from build123d import *

# Parameters (mm, degrees)
F1_W          = 44.45
F1_H          = 31.75
F2_DEPTH      = 6.985
F4_DEPTH      = 44.45
F6_DEPTH      = 15.24
F6_DEPTH_BACK = 15.24
F7_W          = 20
F7_H          = 8.0811108913
F8_DEPTH      = 25.4
F9_R          = 1.6
F10_DEPTH     = 25.4
F11_R         = 1.6
F12_DEPTH     = 5.7
F13_W         = 31.75
F13_H         = 1.5
F14_DEPTH     = 2
F14_TAPER     = 10
F15_F1_R      = 0.254
F15_F2_R      = 0.254
F16_R         = 5.08
F18_R         = 1.27
F19_T1_DEPTH  = 5.24
F19_T3_DEPTH  = 5.24
F19_T5_DEPTH  = 8.89
F19_T7_DEPTH  = 29.21
F19_T9_DEPTH  = 41.91
F19_S13_W     = 1.2954
F19_S13_H     = 1.2954
F19_T14_DEPTH = 1.2954
F19_S19_W     = 1.2954
F19_S19_H     = 1.2954
F19_T20_DEPTH = 1.2954
F19_S25_W     = 1.2954
F19_S25_H     = 1.2954
F19_T26_DEPTH = 1.2954
F19_S31_W     = 1.2954
F19_S31_H     = 1.2954
F19_T32_DEPTH = 1.2954


# Not quite as in the source:
# - a fillet or chamfer that OpenCascade refuses, or shapes differently, is made with other operations: its cross-section is extruded or revolved along the edge and cut away or added
# - a feature of the source that left no trace in its solid (it failed there, or was rolled back) is left out


with BuildPart() as f2:
    # F1 (on Top) → F2 (new body)
    with BuildSketch(Plane.XY):
        Rectangle(F1_W, F1_H)
    extrude(amount=-F2_DEPTH)

    # F3 (on face) → F4 (cut, through all)
    with BuildSketch(Plane.YZ.offset(22.225)):
        with BuildLine():
            add(Edge.make_bspline(
                [(-4.125, 4.125), (-2.4255892558, 4.1137489608), (-0.0276085061, 2.971292738), (2.5249406681, 4.1137612248), (4.191, 4.191)],
                knots=[0, 0, 0, 0, 0.4977710734, 1, 1, 1, 1], degree=3))
            ThreePointArc((-4.125, 4.125), (-7.0418154724, 2.9168154724), (-8.25, 0))
            ThreePointArc((-8.25, 0), (-7.0418154724, -2.9168154724), (-4.125, -4.125))
            add(Edge.make_bspline(
                [(-4.125, -4.125), (-2.9335741419, -4.2006121948), (0.4172014685, -3.0581585459), (2.1438994445, -4.2006121948), (4.191, -4.191)],
                knots=[0, 0, 0, 0, 0.497799261, 1, 1, 1, 1], degree=3))
            ThreePointArc((4.191, -4.191), (7.15448452, -2.96348452), (8.382, 0))
            ThreePointArc((8.382, 0), (7.15448452, 2.96348452), (4.191, 4.191))
        make_face()
    extrude(amount=-F4_DEPTH, mode=Mode.SUBTRACT)

    # F5 (on Right) → F6 (join, two sides)
    with BuildSketch(Plane.YZ) as f6_sk:
        with BuildLine():
            ThreePointArc((-31.115, -30.5349261659), (0, -16.985), (31.115, -30.5349261659))
            Line((31.115, -30.5349261659), (28.575, -25.0251942949))
            ThreePointArc((28.575, -25.0251942949), (19.6900567688, -18.8213349574), (9.525, -15.0661108913))
            ThreePointArc((9.525, -15.0661108913), (0, -13.985), (-9.525, -15.0661108913))
            ThreePointArc((-9.525, -15.0661108913), (-19.6900567688, -18.8213349574), (-28.575, -25.0251942949))
            Line((-28.575, -25.0251942949), (-31.115, -30.5349261659))
        make_face()
        with BuildLine():
            ThreePointArc((-9.525, -15.0661108913), (0, -13.985), (9.525, -15.0661108913))
            Line((9.525, -15.0661108913), (9.525, -6.985))
            Line((9.525, -6.985), (-9.525, -6.985))
            Line((-9.525, -6.985), (-9.525, -15.0661108913))
        make_face()
    extrude(amount=F6_DEPTH)
    extrude(f6_sk.sketch, amount=-F6_DEPTH_BACK)

    # F7 (on face) → F8 (cut)
    with BuildSketch(Plane.XZ.offset(9.525)):
        with Locations((0, -11.0255554456)):
            Rectangle(F7_W, F7_H)
    extrude(amount=-F8_DEPTH, mode=Mode.SUBTRACT)

    # F9 (on face) → F10 (cut)
    with BuildSketch(Plane(origin=(0, 0, -6.985), x_dir=(1, 0, 0), z_dir=(0, 0, -1))):
        with Locations((-18.669, 12.319)):
            Circle(F9_R)
        with Locations((18.669, -12.319)):
            Circle(F9_R)
    extrude(amount=-F10_DEPTH, mode=Mode.SUBTRACT)

    # F11 (on face) → F12 (cut)
    with BuildSketch(Plane(origin=(0, 0, -6.985), x_dir=(1, 0, 0), z_dir=(0, 0, -1))):
        Polygon((-17.344, 10.02403268), (-16.019, 12.319), (-17.344, 14.61396732), (-19.994, 14.61396732), (-21.319, 12.319), (-19.994, 10.02403268), align=None)
        with Locations((-18.669, 12.319)):
            Circle(F11_R, mode=Mode.SUBTRACT)
        Polygon((19.994, -14.61396732), (21.319, -12.319), (19.994, -10.02403268), (17.344, -10.02403268), (16.019, -12.319), (17.344, -14.61396732), align=None)
        with Locations((18.669, -12.319)):
            Circle(F11_R, mode=Mode.SUBTRACT)
    extrude(amount=-F12_DEPTH, mode=Mode.SUBTRACT)

    # F13 (on face) → F14 (join)
    with BuildSketch(Plane.XY):
        with Locations((-4.35, 13.125)):
            Rectangle(F13_W, F13_H)
        with Locations((4.35, -13.125)):
            Rectangle(F13_W, F13_H)
    extrude(amount=F14_DEPTH, taper=F14_TAPER)

    # F15: fillet of radius 0.254 on 2 edges, made by hand

    # F15_f1
    f15_f1_edges = [f2.edges().sort_by_distance(p)[0] for p in [
        (0, -31.115, -30.5349261659),
    ]]
    fillet(f15_f1_edges, radius=F15_F1_R)

    # F15_f2
    f15_f2_edges = [f2.edges().sort_by_distance(p)[0] for p in [
        (0, 31.115, -30.5349261659),
    ]]
    fillet(f15_f2_edges, radius=F15_F2_R)

    # F16
    f16_edges = [f2.edges().sort_by_distance(p)[0] for p in [
        (0, 28.575, -25.025194),
        (0, -28.575, -25.025194),
    ]]
    fillet(f16_edges, radius=F16_R)

    # F18
    f18_edges = [f2.edges().sort_by_distance(p)[0] for p in [
        (12.62, 9.525, -6.985),
        (15.24, 0, -6.985),
        (12.62, -9.525, -6.985),
        (10, 0, -6.985),
        (-12.62, -9.525, -6.985),
        (-15.24, 0, -6.985),
        (-10, 0, -6.985),
        (-12.62, 9.525, -6.985),
    ]]
    fillet(f18_edges, radius=F18_R)

    # F19: fillet of radius 1.27 on 12 edges, made by hand

    # F19_s2 → F19_t1 (join)
    with BuildSketch(Plane.YZ.offset(-15.24)):
        with BuildLine():
            ThreePointArc((9.525, -14.0670689448), (9.7923311345, -14.8465271838), (10.4817797578, -15.2978382489))
            ThreePointArc((10.4817797578, -15.2978382489), (10.0040608486, -15.1792042016), (9.525, -15.0661108913))
            Line((9.525, -15.0661108913), (9.525, -14.0670689448))
        make_face()
        with BuildLine():
            ThreePointArc((-9.525, -14.0670689448), (-9.7923311345, -14.8465271838), (-10.4817797578, -15.2978382489))
            ThreePointArc((-10.4817797578, -15.2978382489), (-10.0040608486, -15.1792042016), (-9.525, -15.0661108913))
            Line((-9.525, -15.0661108913), (-9.525, -14.0670689448))
        make_face()
    extrude(amount=F19_T1_DEPTH)

    # F19_s4 → F19_t3 (join)
    with BuildSketch(Plane.YZ.offset(10)):
        with BuildLine():
            ThreePointArc((10.4817797578, -15.2978382489), (9.7923311345, -14.8465271838), (9.525, -14.0670689448))
            Line((9.525, -14.0670689448), (9.525, -15.0661108913))
            ThreePointArc((9.525, -15.0661108913), (10.0040608486, -15.1792042016), (10.4817797578, -15.2978382489))
        make_face()
        with BuildLine():
            ThreePointArc((-10.4817797578, -15.2978382489), (-9.7923311345, -14.8465271838), (-9.525, -14.0670689448))
            Line((-9.525, -14.0670689448), (-9.525, -15.0661108913))
            ThreePointArc((-9.525, -15.0661108913), (-10.0040608486, -15.1792042016), (-10.4817797578, -15.2978382489))
        make_face()
    extrude(amount=F19_T3_DEPTH)

    # F19_s6 → F19_t5 (cut)
    with BuildSketch(Plane.XY.offset(-5.715)):
        with BuildLine():
            ThreePointArc((-20.955, -15.875), (-21.8530256121, -15.5030256121), (-22.225, -14.605))
            Line((-22.225, -14.605), (-22.225, -15.875))
            Line((-22.225, -15.875), (-20.955, -15.875))
        make_face()
        with BuildLine():
            ThreePointArc((22.225, -14.605), (21.8530256121, -15.5030256121), (20.955, -15.875))
            Line((20.955, -15.875), (22.225, -15.875))
            Line((22.225, -15.875), (22.225, -14.605))
        make_face()
        with BuildLine():
            ThreePointArc((22.225, 14.605), (21.8530256121, 15.5030256121), (20.955, 15.875))
            Line((20.955, 15.875), (22.225, 15.875))
            Line((22.225, 15.875), (22.225, 14.605))
        make_face()
        with BuildLine():
            ThreePointArc((-20.955, 15.875), (-21.8530256121, 15.5030256121), (-22.225, 14.605))
            Line((-22.225, 14.605), (-22.225, 15.875))
            Line((-22.225, 15.875), (-20.955, 15.875))
        make_face()
    extrude(amount=F19_T5_DEPTH, mode=Mode.SUBTRACT)

    # F19_s8 → F19_t7 (cut)
    with BuildSketch(Plane.XZ.offset(-14.605)):
        with BuildLine():
            ThreePointArc((-20.955, -6.985), (-21.8530256121, -6.6130256121), (-22.225, -5.715))
            Line((-22.225, -5.715), (-22.225, -6.985))
            Line((-22.225, -6.985), (-20.955, -6.985))
        make_face()
        with BuildLine():
            ThreePointArc((20.955, -6.985), (21.8530256121, -6.6130256121), (22.225, -5.715))
            Line((22.225, -5.715), (22.225, -6.985))
            Line((22.225, -6.985), (20.955, -6.985))
        make_face()
    extrude(amount=F19_T7_DEPTH, mode=Mode.SUBTRACT)

    # F19_s10 → F19_t9 (cut)
    with BuildSketch(Plane.YZ.offset(-20.955)):
        with BuildLine():
            ThreePointArc((-14.605, -6.985), (-15.5030256121, -6.6130256121), (-15.875, -5.715))
            Line((-15.875, -5.715), (-15.875, -6.985))
            Line((-15.875, -6.985), (-14.605, -6.985))
        make_face()
        with BuildLine():
            ThreePointArc((14.605, -6.985), (15.5030256121, -6.6130256121), (15.875, -5.715))
            Line((15.875, -5.715), (15.875, -6.985))
            Line((15.875, -6.985), (14.605, -6.985))
        make_face()
    extrude(amount=F19_T9_DEPTH, mode=Mode.SUBTRACT)


with BuildPart() as f19_tool12:
    # F19_s13 → F19_t14 (new body)
    with BuildSketch(Plane.YZ.offset(-20.955)):
        with Locations((-15.2527, -6.3627)):
            Rectangle(F19_S13_W, F19_S13_H)
    extrude(amount=-F19_T14_DEPTH)

    # F19_s15 → F19_t16 (revolve, cut)
    with BuildSketch(Plane(origin=(-20.955, -14.605, -5.715), x_dir=(0, 0.7071067812, 0.7071067812), z_dir=(0, -0.7071067812, 0.7071067812))):
        with BuildLine():
            ThreePointArc((0, -1.27), (1.27, 0), (0, 1.27))
            Line((0, 1.27), (0, -1.27))
        make_face()
    revolve(axis=Axis((-20.955, -14.605, -5.715), (-1, 0, 0)), mode=Mode.SUBTRACT)


with BuildPart() as f2_1:
    add(f2.part)

    # F19_t11: cut F19_tool12
    add(f19_tool12.part, mode=Mode.SUBTRACT)


with BuildPart() as f19_tool18:
    # F19_s19 → F19_t20 (new body)
    with BuildSketch(Plane.XY.offset(-5.715)):
        with Locations((-21.6027, 15.2527)):
            Rectangle(F19_S19_W, F19_S19_H)
    extrude(amount=-F19_T20_DEPTH)

    # F19_s21 → F19_t22 (revolve, cut)
    with BuildSketch(Plane(origin=(-20.955, 14.605, -5.715), x_dir=(0.7071067812, -0.7071067812, 0), z_dir=(0.7071067812, 0.7071067812, 0))):
        with BuildLine():
            ThreePointArc((0, -1.27), (1.27, 0), (0, 1.27))
            Line((0, 1.27), (0, -1.27))
        make_face()
    revolve(axis=Axis((-20.955, 14.605, -5.715), (0, 0, -1)), mode=Mode.SUBTRACT)


with BuildPart() as f2_2:
    add(f2_1.part)

    # F19_t17: cut F19_tool18
    add(f19_tool18.part, mode=Mode.SUBTRACT)


with BuildPart() as f19_tool24:
    # F19_s25 → F19_t26 (new body)
    with BuildSketch(Plane.XY.offset(-5.715)):
        with Locations((21.6027, -15.2527)):
            Rectangle(F19_S25_W, F19_S25_H)
    extrude(amount=-F19_T26_DEPTH)

    # F19_s27 → F19_t28 (revolve, cut)
    with BuildSketch(Plane(origin=(20.955, -14.605, -5.715), x_dir=(-0.7071067812, 0.7071067812, 0), z_dir=(-0.7071067812, -0.7071067812, 0))):
        with BuildLine():
            ThreePointArc((0, -1.27), (1.27, 0), (0, 1.27))
            Line((0, 1.27), (0, -1.27))
        make_face()
    revolve(axis=Axis((20.955, -14.605, -5.715), (0, 0, -1)), mode=Mode.SUBTRACT)


with BuildPart() as f2_3:
    add(f2_2.part)

    # F19_t23: cut F19_tool24
    add(f19_tool24.part, mode=Mode.SUBTRACT)


with BuildPart() as f19_tool30:
    # F19_s31 → F19_t32 (new body)
    with BuildSketch(Plane.XY.offset(-5.715)):
        with Locations((21.6027, 15.2527)):
            Rectangle(F19_S31_W, F19_S31_H)
    extrude(amount=-F19_T32_DEPTH)

    # F19_s33 → F19_t34 (revolve, cut)
    with BuildSketch(Plane(origin=(20.955, 14.605, -5.715), x_dir=(-0.7071067812, -0.7071067812, 0), z_dir=(0.7071067812, -0.7071067812, 0))):
        with BuildLine():
            ThreePointArc((0, -1.27), (1.27, 0), (0, 1.27))
            Line((0, 1.27), (0, -1.27))
        make_face()
    revolve(axis=Axis((20.955, 14.605, -5.715), (0, 0, -1)), mode=Mode.SUBTRACT)


with BuildPart() as f2_4:
    add(f2_3.part)

    # F19_t29: cut F19_tool30
    add(f19_tool30.part, mode=Mode.SUBTRACT)


solid = f2_4.part
Could you check a few things on this model? Use its own coordinates, in mm. A direction names the side the tool comes from. Round coordinates to 2 decimals unless told otherwise and drop trailing zeros. Order: outer loops, then holes, each group sorted by start corner. A loop starts at its lowest first (then second) coordinate and runs counter-clockwise, first axis right, second up. Notation, with made-up numbers: M 13,82 L 64,82 A15 ccw 64,89 Z; hole C 33.5,-21.75 d11. An arc over 180 degrees is marked long. One line per item, written item: value.
(1) Imagine slicing it at A-A (z = -11). Write out the boundary of the cut face in (x, y) (3 decimals).
Ans:
outline: M -15.24,-9.525 L -10,-9.525 L -10,9.525 L -15.24,9.525 Z; M 10,-9.525 L 15.24,-9.525 L 15.24,9.525 L 10,9.525 Z
(2) I need wall thicknesses on line 1 along X through (y, z) = (-18.5, -20); line 2 along Y through (x, z) = (6.5, -21); line 3 along X through (y, z) = (4, -8). Which ranges of each line are inside material? Lowest first, please. Write a range as from..to.
Ans:
line 1: x = -15.24..15.24
line 2: y = -23.39..-18.03, 18.03..23.39
line 3: x = -15.27..-9.97, 9.97..15.27
(3) Which directions (+Z, -Z, +X, -X, +Y, -Y) give clear straight access to the entire face, cutting with the end or side of a thin tool? Please do faces 1 (the cylindrical face through (-12.657, -9.785, -14.837)), 2 (the flat face through (15.24, 0, -16)), 3 (the cylindrical face through (0.31, 7.12, -3)), 4 (the flat face through (0, 0, -15.066)), 5 (the flat face through (-19, -14.614, -4)).
Ans:
face 1: +X, -X, -Y
face 2: -Z, +X, +Y, -Y
face 3: +Z, +X, -X
face 4: +Y, -Y
face 5: -Z
(4) Imagine slicing it at B-B (z = -2.5). Write out the boundary of the cut face in (x, y) (3 decimals).
Ans:
outline: M -22.225,-14.605 A1.27 ccw -20.955,-15.875 L 20.955,-15.875 A1.27 ccw 22.225,-14.605 L 22.225,-7.406 L -22.225,-7.406 Z; M -22.225,7.555 L 22.225,7.555 L 22.225,14.605 A1.27 ccw 20.955,15.875 L -20.955,15.875 A1.27 ccw -22.225,14.605 Z; hole M -21.319,-12.319 L -19.994,-14.614 L -17.344,-14.614 L -16.019,-12.319 L -17.344,-10.024 L -19.994,-10.024 Z; hole M 16.019,12.319 L 17.344,10.024 L 19.994,10.024 L 21.319,12.319 L 19.994,14.614 L 17.344,14.614 Z
(5) I'm going to push flat-ended pins straight in: P1, Ø14.5, axis at x = -7, y = 3.5, coming from the -Z side; P2, Ø2, axis at x = -19, z = -3.5, coming from the -Y side (3 decimals); P3, Ø8, axis at x = -12.5, y = 24, coming from the +Z side (3 decimals); P4, Ø2, axis at y = -1, z = -19, coming from the -X side. Where does each tip first touch, or does it pass through?
Ans:
P1: stops at z = -18.37
P2: stops at y = -15.875
P3: stops at z = -18.985
P4: passes through
(6) Imagine slicing it at C-C (y = -5.5). Write out the boundary of the cut face in (x, z) (3 decimals).
Ans:
outline: M -22.225,-5.715 A1.27 ccw -20.955,-6.985 L -16.51,-6.985 A1.27 cw -15.24,-8.255 L -15.24,-17.342 L 15.24,-17.342 L 15.24,-8.255 A1.27 cw 16.51,-6.985 L 20.955,-6.985 A1.27 ccw 22.225,-5.715 L 22.225,-3.889 L -22.225,-3.889 Z; hole M -10,-15.066 L 10,-15.066 L 10,-8.255 A1.27 ccw 8.73,-6.985 L -8.73,-6.985 A1.27 ccw -10,-8.255 Z
(7) If we mould it in two halves opening along Z, with no side actions, what happens to faces 6 (the flat face through (-16.7, -13.5, -4.2)), 7 (the flat face through (0.213, 29.764, -27.605)), 8 (the cylindrical face through (12.583, 9.8, -14.856))? For each: released by +Z, released by -Z, zero draft, split by the parting line, or undercut.
Ans:
face 6: zero draft
face 7: released by +Z
face 8: undercut
(8) Imagine slicing it at D-D (z = -22.5). Write out the boundary of the cut face in (x, y), and give its area (3 significant figures).
Ans:
outline: M -15.24,-25.52 L 15.24,-25.52 L 15.24,-20.94 L -15.24,-20.94 Z; M -15.24,20.94 L 15.24,20.94 L 15.24,25.52 L -15.24,25.52 Z
area: 279 mm^2
